Answer from the drawing. Dimensions are ordinates in mm from the lowest x, y and z of the part. A direction names the side the tool comes from. Coordinates: 2 decimals unless noted, no trailing zeros. Loops run counter-clockwise (first coordinate to the right, second up) from the corner with the lowest first, then second, coordinate; pieces in that order, holes last. Notation, with made-up numbers: (-26, 29.25) - (-15, 29.25) arc R14 cw to (-15, 47.25) - close; hole circle Ø11 at (78, 37). An arc over 180 degrees is marked (long way). Use one line per item in the form item = value. Start each with the question number.
1) A cutting plane is placed at B-B (x = 42.4). Give the vertices of the cut face in (y, z).
2) A cutting plane is placed at D-D (y = 9). Give the vertices of the cut face in (x, z), and give its area (3 significant figures).
3) Each of these flat-tipped pins is pushed along its axis until it touches: P1, Ø9, axis at x = 42.4, z = 12.7, coming from the +Y side; P2, Ø8, axis at x = 25.4, z = 12.7, coming from the -Y side. Where does it stop, or does it pass through?
4) Consider line 1 (X direction, y = 7.75, z = 12.5); line 2 (X direction, y = 6, z = 9.75); line 3 (Y direction, x = 42.5, z = 7.5). Determine where each line is inside the solid, lowest interval first.
5) The mould has two halves that part along Z. Classify the marked faces 1, 2, 3 and 4: released by +Z, released by -Z, zero draft, split by the parting line, or undercut.
6) Which of the six approach directions +Z, -Z, +X, -X, +Y, -Y give full straight-line access (tool end or side, diameter ignored) to the marked faces 5 and 6?
7) A cutting plane is placed at C-C (z = 12.7). Give the vertices of the cut face in (x, y).
8) A cutting plane is placed at A-A (y = 3). Give the vertices of the cut face in (x, z).
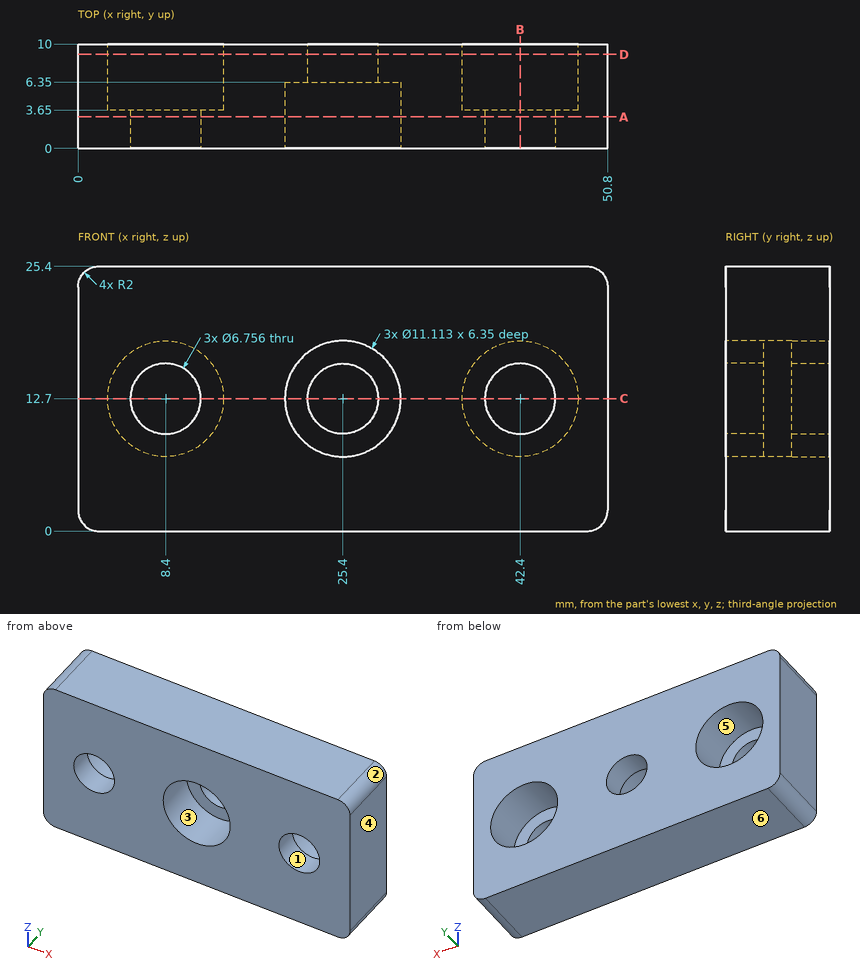
Found:
q1.outline = (0, 0) - (10, 0) - (10, 7.14) - (3.65, 7.14) - (3.65, 9.32) - (0, 9.32) - close; (0, 16.08) - (3.65, 16.08) - (3.65, 18.26) - (10, 18.26) - (10, 25.4) - (0, 25.4) - close
q2.outline = (0, 2) arc R2 ccw to (2, 0) - (48.8, 0) arc R2 ccw to (50.8, 2) - (50.8, 23.4) arc R2 ccw to (48.8, 25.4) - (2, 25.4) arc R2 ccw to (0, 23.4) - close; hole circle Ø11.11 at (8.4, 12.7); hole circle Ø6.76 at (25.4, 12.7); hole circle Ø11.11 at (42.4, 12.7)
q2.area = 1,060 mm^2
q3.P1 = 3.65
q3.P2 = 6.35
q4.line_1 = 0 to 2.85, 13.95 to 22.03, 28.77 to 36.85, 47.95 to 50.8
q4.line_2 = 0 to 3.69, 13.11 to 20.69, 30.11 to 37.69, 47.11 to 50.8
q4.line_3 = 0 to 3.65
q5.face_1 = undercut
q5.face_2 = released by +Z
q5.face_3 = undercut
q5.face_4 = zero draft
q6.face_5 = +Y
q6.face_6 = -Z, +X, -X, +Y, -Y
q7.outline = (0, 0) - (5.02, 0) - (5.02, 3.65) - (2.84, 3.65) - (2.84, 10) - (0, 10) - close; (11.78, 0) - (19.84, 0) - (19.84, 6.35) - (22.02, 6.35) - (22.02, 10) - (13.96, 10) - (13.96, 3.65) - (11.78, 3.65) - close; (28.78, 6.35) - (30.96, 6.35) - (30.96, 0) - (39.02, 0) - (39.02, 3.65) - (36.84, 3.65) - (36.84, 10) - (28.78, 10) - close; (45.78, 0) - (50.8, 0) - (50.8, 10) - (47.96, 10) - (47.96, 3.65) - (45.78, 3.65) - close
q8.outline = (0, 2) arc R2 ccw to (2, 0) - (48.8, 0) arc R2 ccw to (50.8, 2) - (50.8, 23.4) arc R2 ccw to (48.8, 25.4) - (2, 25.4) arc R2 ccw to (0, 23.4) - close; hole circle Ø6.76 at (8.4, 12.7); hole circle Ø11.11 at (25.4, 12.7); hole circle Ø6.76 at (42.4, 12.7)
